Part model, mm, in its own coordinate system. Coordinates: 2 decimals unless noted, no trailing zeros. Write each loop counter-clockwise with the first axis right and the second up, starting at its lowest first coordinate (ties: lowest second). Pieces come first, ordered by that corner, then holes. Notation, with made-up numbers: (59.25, 34.5) -> (78.25, 34.5) arc R18 ccw to (78.25, 68.5) -> close; hole circle Ø11 at (67.5, 64). An arc over 180 degrees is marked (long way). One line per question, with ' | ' between items. Start each with the question number.
Item 1: Saw through at A-A (z = 39). List the corners of the cut face in (x, y), and give its area (3 significant figures).
Item 2: Pin check, flat tips, straight feed: pin 1 (6 mm diameter, centred on x = -3.5, z = 21, fed in from +Y); pin 2 (0.5 mm diameter, centred on x = -1, y = -12.5, fed in from -Z); pin 3 (5 mm diameter, centred on y = -12, z = 26, fed in from -X). Stop position of each tip, or through.
Item 3: Probe probe 1 along Z at (x, y) = (6, 5); probe 2 along Y at (x, z) = (2.5, 7.5); probe 3 along X at (y, z) = (-12, 5). List the from-to ranges inside material, lowest first. Write a range as [from, to].
Item 4: Saw through at B-B (z = 6). List the corners of the cut face in (x, y).
from build123d import *

# Parameters (mm, degrees)
SKETCH1_R           = 9.75
SKETCH1_R_2         = 0.5
BOSS_EXTRUDE1_DEPTH = 2
SKETCH3_R           = 10
BOSS_EXTRUDE2_DEPTH = 48
BOSS_EXTRUDE2_TAPER = 10
BOSS_EXTRUDE3_DEPTH = 5
SKETCH5_W           = 5
SKETCH5_H           = 5
BOSS_EXTRUDE4_DEPTH = 6


with BuildPart() as part:
    # Sketch1 → Boss-Extrude1 (new body)
    with BuildSketch(Plane.XY):
        with Locations((4.234062462, -7.179497219)):
            Circle(SKETCH1_R)
        with Locations((4.234062462, 0.270502781)):
            Circle(SKETCH1_R_2, mode=Mode.SUBTRACT)
        with Locations((9.502007982, -1.911551699)):
            Circle(SKETCH1_R_2, mode=Mode.SUBTRACT)
        with Locations((11.684062462, -7.179497219)):
            Circle(SKETCH1_R_2, mode=Mode.SUBTRACT)
        with Locations((9.502007982, -12.447442738)):
            Circle(SKETCH1_R_2, mode=Mode.SUBTRACT)
        with Locations((4.234062462, -14.629497219)):
            Circle(SKETCH1_R_2, mode=Mode.SUBTRACT)
        with Locations((-1.033883058, -12.447442738)):
            Circle(SKETCH1_R_2, mode=Mode.SUBTRACT)
        with Locations((-3.215937538, -7.179497219)):
            Circle(SKETCH1_R_2, mode=Mode.SUBTRACT)
        with Locations((-1.033883058, -1.911551699)):
            Circle(SKETCH1_R_2, mode=Mode.SUBTRACT)
    extrude(amount=BOSS_EXTRUDE1_DEPTH)

    # Sketch3 → Boss-Extrude2 (add)
    with BuildSketch(Plane.XY.offset(2)):
        with Locations((4.234062462, -7.179497219)):
            Circle(SKETCH3_R)
    extrude(amount=BOSS_EXTRUDE2_DEPTH, taper=BOSS_EXTRUDE2_TAPER)

    # Sketch4 → Boss-Extrude3 (add)
    with BuildSketch(Plane(origin=(0, 0, 0), x_dir=(-1, 0, 0), z_dir=(0, 0, -1))):
        with BuildLine():
            ThreePointArc((-6.734062462, 2.244541194), (-5.494642781, 2.48866896), (-4.234062462, 2.570502781))
            Line((-4.234062462, 2.570502781), (-4.234062462, 7.570502781))
            Line((-4.234062462, 7.570502781), (-6.734062462, 7.570502781))
            Line((-6.734062462, 7.570502781), (-6.734062462, 2.244541194))
        make_face()
        with BuildLine():
            Line((-4.234062462, 7.570502781), (-4.234062462, 2.570502781))
            ThreePointArc((-4.234062462, 2.570502781), (-2.973482144, 2.48866896), (-1.734062462, 2.244541194))
            Line((-1.734062462, 2.244541194), (-1.734062462, 7.570502781))
            Line((-1.734062462, 7.570502781), (-4.234062462, 7.570502781))
        make_face()
    extrude(amount=-BOSS_EXTRUDE3_DEPTH)

    # Sketch5 → Boss-Extrude4 (add)
    with BuildSketch(Plane(origin=(0, 7.570502781, 0), x_dir=(1, 0, 0), z_dir=(0, 1, 0))):
        with Locations((4.234062462, -2.5)):
            Rectangle(SKETCH5_W, SKETCH5_H)
    extrude(amount=-BOSS_EXTRUDE4_DEPTH)


solid = part.part
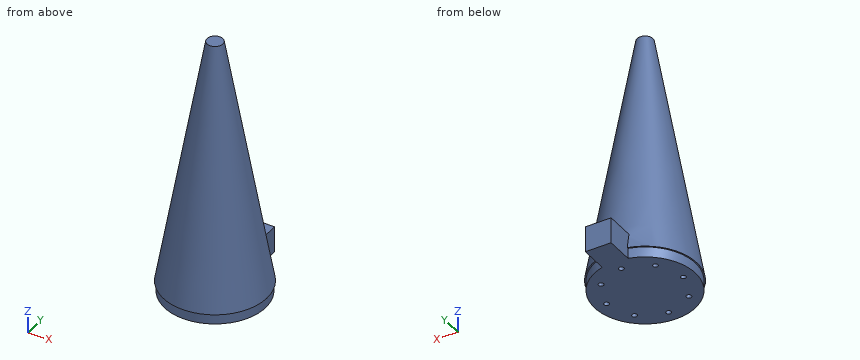
From the geometry:
1) outline: circle Ø6.95 at (4.23, -7.18) | area: 38.0 mm2
2) pin 1: y = -2.42 | pin 2: z = 2 | pin 3: x = -1.15
3) probe 1: [0, 5] | probe 2: [-16.04, 1.68] | probe 3: [-3.92, 12.39]
4) outline: circle Ø18.59 at (4.23, -7.18)
